```python
from build123d import *

# Parameters (mm, degrees)
F_6_32_TAPPED_HOLE1_AT_2_COUNT = 2
F_6_32_TAPPED_HOLE1_AT_2_PITCH = 11.313708499
F_6_32_TAPPED_HOLE1_AT_3_COUNT = 2
F_6_32_TAPPED_HOLE1_AT_3_PITCH = 11.313708499
F_6_32_TAPPED_HOLE1_AT_4_COUNT = 2
F_6_32_TAPPED_HOLE1_AT_4_PITCH = 16
BOSS_EXTRUDE1_START            = 10
SKETCH4_R                      = 1.25
BOSS_EXTRUDE1_DEPTH            = 1.5
F_8_32_TAPPED_HOLE1_D          = 3.4544
F_8_32_TAPPED_HOLE1_DEPTH      = 10.708
F_8_32_TAPPED_HOLE1_TIP        = 1.037806461
CHAMFER1_SIZE                  = 0.3


with BuildPart() as part:
    # Sketch1 → Revolve1 (revolve)
    with BuildSketch(Plane.XY):
        Polygon((-9.5, 3), (2.5, 3), (2.5, 4), (0, 4), (0, 14.2621), (-2.5, 14.2621), (-2.5, 11.5), (-9.5, 11.5), align=None)
    revolve(axis=Axis((0, 0, 0), (1, 0, 0)))

    # Sketch3 → 6-32 Tapped Hole1 (revolve, cut)
    with BuildSketch(Plane(origin=(0, 0, 8), x_dir=(0, 0, -1), z_dir=(0, 1, 0))):
        Polygon((0, 0), (0, 9.5), (1.98755, 9.5), (1.35255, 8.865), (1.35255, 0.635), (1.98755, 0), align=None)
    f_6_32_tapped_hole1 = revolve(axis=Axis((6.35, 0, 8), (-1, 0, 0)), mode=Mode.SUBTRACT)

    # 6-32 Tapped Hole1 at 2: 6-32 Tapped Hole1 ×2
    with Locations(*[Vector(0, 0.707106781, -0.707106781) * (i * F_6_32_TAPPED_HOLE1_AT_2_PITCH) for i in range(1, F_6_32_TAPPED_HOLE1_AT_2_COUNT)]):
        add(f_6_32_tapped_hole1, mode=Mode.SUBTRACT)

    # 6-32 Tapped Hole1 at 3: 6-32 Tapped Hole1 ×2
    with Locations(*[Vector(0, -0.707106781, -0.707106781) * (i * F_6_32_TAPPED_HOLE1_AT_3_PITCH) for i in range(1, F_6_32_TAPPED_HOLE1_AT_3_COUNT)]):
        add(f_6_32_tapped_hole1, mode=Mode.SUBTRACT)

    # 6-32 Tapped Hole1 at 4: 6-32 Tapped Hole1 ×2
    with Locations(*[(0, 0, -i * F_6_32_TAPPED_HOLE1_AT_4_PITCH) for i in range(1, F_6_32_TAPPED_HOLE1_AT_4_COUNT)]):
        add(f_6_32_tapped_hole1, mode=Mode.SUBTRACT)

    # Sketch4 → Boss-Extrude1 (add)
    with BuildSketch(Plane(origin=(0, 0, 0), x_dir=(-1, 0, 0), z_dir=(0, 0.707106781, 0.707106781)).offset(BOSS_EXTRUDE1_START)):
        with Locations((6, 0)):
            Circle(SKETCH4_R)
    extrude(amount=BOSS_EXTRUDE1_DEPTH)

    # 8-32 Tapped Hole1
    with Locations(Plane(origin=(0, 8.131727984, 8.131727984), x_dir=(1, 0, 0), z_dir=(0, 0.707106781, 0.707106781))):
        with Locations((-6, 0)):
            Hole(F_8_32_TAPPED_HOLE1_D / 2, depth=F_8_32_TAPPED_HOLE1_DEPTH)
            with Locations((0, 0, -(F_8_32_TAPPED_HOLE1_DEPTH + F_8_32_TAPPED_HOLE1_TIP / 2))):  # 118° drill point
                Cone(0, F_8_32_TAPPED_HOLE1_D / 2, F_8_32_TAPPED_HOLE1_TIP, mode=Mode.SUBTRACT)

    # Chamfer1
    chamfer1_edges = [part.edges().sort_by_distance(p)[0] for p in [
        (-9.5, -3, 0),
        (2.5, -3, 0),
        (2.5, -4, 0),
        (0, -14.2621, 0),
        (-2.5, -14.2621, 0),
        (-9.5, -11.5, 0),
    ]]
    chamfer(chamfer1_edges, length=CHAMFER1_SIZE)


solid = part.part
```
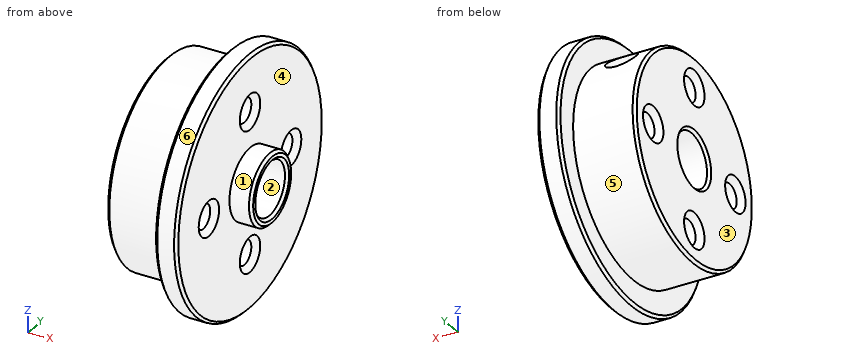
Geometry: final body of the model. Coordinates: model frame, mm. Face numbers are marked on the shaded views. A direction names the side the tool comes from. Round coordinates to 2 decimals unless told otherwise and drop trailing zeros. Write each loop counter-clockwise with the first axis right and the second up, starting at its lowest first coordinate (ties: lowest second). Pieces come first, ordered by that corner, then holes. Notation, with made-up numbers: M -31.75,-5 L 1.25,-5 A32 ccw 1.25,25 Z; hole C -13,58.25 d2. An arc over 180 degrees is marked long. Answer in a Markdown table with one row per item. Add a question column.
(1) Reachability of the marked faces 4, 5 and 6 from +Z, -Z, +X, -X, +Y, -Y: full face, straight path, thin tool, end or side. Return the list, or none.
(2) Cut plane A-A, the plane x = -3.5. Return the cut outline in (y, z), then the cut area to 3 significant figures.
(3) Cut plane C-C, the plane y = 0. Give the number of separate pieces and of enclosed holes in the cut face, then the cut area to 3 significant figures.
(4) Draft query along Y for the marked faces 1, 2 and 3. Return one class per face: pulls with the +Y half, pulls with the -Y half, needs draft (parallel to the pull), parting line crosses it, or undercut.
(5) Cut plane B-B, the plane x = 1.5. Return the cut outline in (y, z).
(6) Contact query for flat-ended pins moving along their axis: pin 1 (1 mm diameter, centred on x = -8, z = -6.5, fed in from +Y); pin 2 (14 mm diameter, centred on y = 6.5, z = -5.5, fed in from +X); pin 3 (3.5 mm diameter, centred on y = 8, z = 0, fed in from -X); pin 4 (1.6 mm diameter, centred on y = -8, z = 0, fed in from +X) (1 decimal). Output: stop coordinate, or through.
(7) Ray query, L1, parallel to Z at x = -4, y = 0; L2, parallel to X at y = 9.5, z = 8; L3, parallel to X at y = -2.5, z = -9.5. Return the intervals inside material, ascending.
Established:
| question | item | result |
|---|---|---|
| 1 | face 4 | +X |
| 1 | face 5 | -X |
| 1 | face 6 | +X, -X |
| 2 | outline | C 0,0 d23; hole C -8,0 d2.71; hole C 0,0 d6; hole C 0,-8 d2.71; hole C 0,8 d2.71; hole C 8,0 d2.71 |
| 2 | area | 364 mm² |
| 3 | separate pieces | 4 |
| 3 | enclosed holes | 0 |
| 3 | area | 127 mm² |
| 4 | face 1 | parting line crosses it |
| 4 | face 2 | undercut |
| 4 | face 3 | needs draft |
| 5 | outline | C 0,0 d8; hole C 0,0 d6 |
| 6 | pin 1 | y = 9.81 |
| 6 | pin 2 | x = 2.5 |
| 6 | pin 3 | x = -9.26 |
| 6 | pin 4 | through |
| 7 | L1 | -11.5 to -9.35, -6.65 to -3, 3 to 6.65, 9.35 to 11.5 |
| 7 | L2 | -2.5 to 0 |
| 7 | L3 | -9.5 to 0 |
